from build123d import *

# Parameters (mm, degrees)
SKETCH1_R           = 1.647641354
BOSS_EXTRUDE1_DEPTH = 2.9718
SKETCH2_R           = 1.5875
CUT_EXTRUDE1_DEPTH  = 3.9718


with BuildPart() as part:
    # Sketch1 → Boss-Extrude1 (new body)
    with BuildSketch(Plane(origin=(0, 0, 0), x_dir=(1, 0, 0), z_dir=(0, 1, 0))):
        Polygon((-17.417287452, 11.099582129), (-31.75, 11.099582129), (-31.75, 4.775417871), (-34.7218, 4.775417871), (-34.7218, -7.924582129), (-31.75, -7.924582129), (-31.75, -20.624582129), (-34.7218, -20.624582129), (-34.7218, -33.324582129), (-31.75, -33.324582129), (-31.75, -36.499582129), (-19.05, -36.499582129), (-19.05, -23.799582129), (19.05, -23.799582129), (19.05, -36.499582129), (31.75, -36.499582129), (31.75, -33.324582129), (34.7218, -33.324582129), (34.7218, -20.624582129), (31.75, -20.624582129), (31.75, -7.924582129), (34.7218, -7.924582129), (34.7218, 4.775417871), (31.75, 4.775417871), (31.75, 11.099582129), (17.417287452, 11.099582129), (17.417287452, -11.099582129), (-17.417287452, -11.099582129), align=None)
        with Locations((-22.179787452, -6.337082129)):
            Circle(SKETCH1_R, mode=Mode.SUBTRACT)
        with Locations((-22.179787452, 6.337082129)):
            Circle(SKETCH1_R, mode=Mode.SUBTRACT)
        with Locations((22.179787452, 6.337082129)):
            Circle(SKETCH1_R, mode=Mode.SUBTRACT)
        with Locations((22.179787452, -6.337082129)):
            Circle(SKETCH1_R, mode=Mode.SUBTRACT)
    extrude(amount=BOSS_EXTRUDE1_DEPTH)

    # Sketch2 → Cut-Extrude1 (cut, through all)
    with BuildSketch(Plane(origin=(0, 2.9718, 0), x_dir=(1, 0, 0), z_dir=(0, 1, 0))):
        with Locations((-33.2359, -1.574582129)):
            Circle(SKETCH2_R)
        with Locations((33.2359, -1.574582129)):
            Circle(SKETCH2_R)
    extrude(amount=-CUT_EXTRUDE1_DEPTH, mode=Mode.SUBTRACT)


solid = part.part
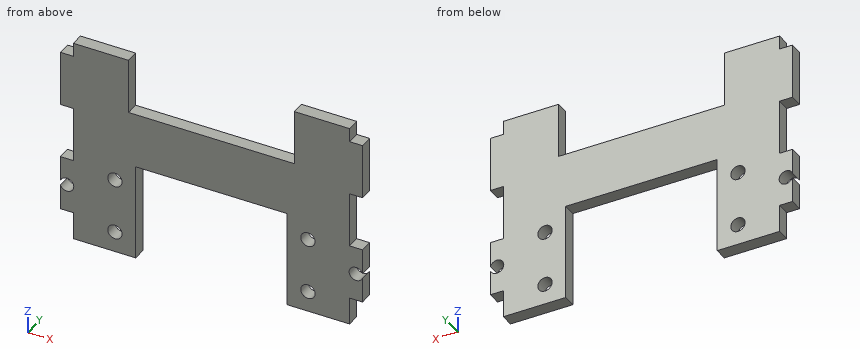
CAD build for the part. Positions are in the model's coordinates, mm. Round coordinates to 2 decimals unless told otherwise and drop trailing zeros. Order: outer loops, then holes, each group sorted by start corner. A loop starts at its lowest first (then second) coordinate and runs counter-clockwise, first axis right, second up. Notation, with made-up numbers: (74.25, 71) - (130.25, 71) arc R8 cw to (130.25, 85) - close; hole circle Ø10 at (9, 55.25). An arc over 180 degrees is marked (long way). Return JSON: item names as keys, results as strings.
(1) Pin check, flat tips, straight feed: pin 1 Ø0.9 at (x, y) = (-33.5, 1.5) entering from +Z; pin 2 Ø0.9 at (x, y) = (-33, 2) entering from -Z; pin 3 Ø0.9 at (y, z) = (1.5, 34) entering from -X. Stop position of each tip, or through.
Answer key:
{"pin 1": "stops at z = 33.32", "pin 2": "stops at z = -4.78", "pin 3": "stops at x = -31.75"}
(2) Cut at B-B (z = -4). Give the cut face in (x, y), then the cut area to 3 significant figures.
Answer key:
{"outline": "(-34.72, 0) - (-17.42, 0) - (-17.42, 2.97) - (-34.72, 2.97) - close; (17.42, 0) - (34.72, 0) - (34.72, 2.97) - (17.42, 2.97) - close", "area": "103 mm^2"}
(3) Cut at A-A (z = 32). Give the cut face in (x, y).
Answer key:
{"outline": "(-34.72, 0) - (-19.05, 0) - (-19.05, 2.97) - (-34.72, 2.97) - close; (19.05, 0) - (34.72, 0) - (34.72, 2.97) - (19.05, 2.97) - close"}
(4) Cut at D-D (y = 1.65). State how many separate pieces and enclosed holes the cut face has, then the cut area to 3 significant figures.
Answer key:
{"separate pieces": "1", "enclosed holes": "4", "area": "1,870 mm^2"}
(5) Cut at C-C (x = 7.5). Give the cut face in (y, z), then the cut area to 3 significant figures.
Answer key:
{"outline": "(0, 11.1) - (2.97, 11.1) - (2.97, 23.8) - (0, 23.8) - close", "area": "37.7 mm^2"}
(6) Wall check: probe 1 along X at (y, z) = (1.7, -4.5); probe 2 along X at (y, z) = (2.4, 25.5); probe 3 along Z at (x, y) = (9, 1.1). Give the ranges that are in metal, low to high. Write a range as from..to.
Answer key:
{"probe 1": "x = -34.72..-17.42, 17.42..34.72", "probe 2": "x = -34.72..-19.05, 19.05..34.72", "probe 3": "z = 11.1..23.8"}
